from build123d import *

# Parameters (mm, degrees)
F0_R     = 1.8
F0_R_2   = 11.25
F1_DEPTH = 3
F2_W     = 60
F2_H     = 5
F3_DEPTH = 17
F4_R     = 1.8
F5_DEPTH = 5.001
F6_R     = 5
F7_R     = 5


with BuildPart() as f1:
    # F0 (on Front) → F1 (new body)
    with BuildSketch(Plane.XZ):
        Polygon((-21, -21), (21, -21), (21, 21), (21, 31), (-21, 31), (-21, 21), align=None)
        with Locations((-15.7, -15.7)):
            Circle(F0_R, mode=Mode.SUBTRACT)
        with Locations((15.7, -15.7)):
            Circle(F0_R, mode=Mode.SUBTRACT)
        Circle(F0_R_2, mode=Mode.SUBTRACT)
        with Locations((-15.7, 15.7)):
            Circle(F0_R, mode=Mode.SUBTRACT)
        with Locations((15.7, 15.7)):
            Circle(F0_R, mode=Mode.SUBTRACT)
    extrude(amount=F1_DEPTH)

    # F2 (on face) → F3 (join)
    with BuildSketch(Plane.XZ.offset(3)):
        with Locations((0, 28.5)):
            Rectangle(F2_W, F2_H)
    extrude(amount=-F3_DEPTH)

    # F4 (on face) → F5 (cut, through all)
    with BuildSketch(Plane(origin=(0, 0, 26), x_dir=(1, 0, 0), z_dir=(0, 0, -1))):
        with Locations((-21.55957, -7)):
            Circle(F4_R)
        with Locations((21.55957, -7)):
            Circle(F4_R)
    extrude(amount=-F5_DEPTH, mode=Mode.SUBTRACT)

    # F6
    f6_edges = [f1.edges().sort_by_distance(p)[0] for p in [
        (21, -1.5, -21),
        (-21, -1.5, -21),
    ]]
    fillet(f6_edges, radius=F6_R)

    # F7
    f7_edges = [f1.edges().sort_by_distance(p)[0] for p in [
        (-30, -3, 28.5),
        (-30, 14, 28.5),
        (30, -3, 28.5),
        (30, 14, 28.5),
    ]]
    fillet(f7_edges, radius=F7_R)


solid = f1.part
Build history of the part. All positions in model axes, mm. A direction names the side the tool comes from. Coordinates: 2 decimals unless noted, no trailing zeros. Order: outer loops, then holes, each group sorted by start corner. A loop starts at its lowest first (then second) coordinate and runs counter-clockwise, first axis right, second up. Notation, with made-up numbers: M -7.5,-4 L 3.5,-4 A17 ccw 3.5,6 Z; hole C -25,85 d2. An arc over 180 degrees is marked long. One line per question, with ' | ' between items. Start each with the question number.
Q1. Probe L1, parallel to Z at x = 15.7, y = -0.9; L2, parallel to X at y = 7, z = 28.65; L3, parallel to Y at x = 7.5, z = -17. List the from-to ranges inside material, lowest first. Write a range as from..to.
Q2. Flat gauge pins, fed straight in: pin 1 Ø4 at (x, z) = (-22, -11) entering from +Y; pin 2 Ø0.9 at (y, z) = (-1, -3) entering from +X; pin 3 Ø0.9 at (y, z) = (-1, 12) entering from -X. Where does each tip first touch, or does it go through?
Q3. Saw through at B-B (x = 0). List the corners of the cut face in (y, z), then the cut area to 4 significant figures.
Q4. Saw through at C-C (z = 4). List the corners of the cut face in (x, y), then the cut area to 3 significant figures.
Q5. Saw through at D-D (x = -6.5). List the corners of the cut face in (y, z).
Q6. Saw through at A-A (z = 15.7). List the corners of the cut face in (x, y), then the cut area to 3 significant figures.
Q7. Two-plate mould, pull along Z, no slides. Class faces 1 (the face through (-17.128, -1.479, -16.795)), 2 (the face through (28, -2, 29)), 3 (the face through (14.373, -1.479, 16.917)), 4 (the face through (0, 7, 26)): +Z half, -Z half, draft (parallel to the pull), parting line (faces both ways), or undercut.
Q8. 3-axis set-ups, long thin cutter, end or side, ignore diameter. For faces 5 (the face through (21, -1, 5)), 6 (the face through (0, 5, 31)), 7 (the face through (-21, -1, 5)): which of +Z, -Z, +X, -X, +Y, -Y reach the whole face in a straight line?
Check values:
1) L1: z = -21..-17.5, -13.9..13.9, 17.5..31 | L2: x = -30..-23.36, -19.76..19.76, 23.36..30 | L3: y = -3..0
2) pin 1: stops at y = 0 | pin 2: stops at x = 21 | pin 3: stops at x = -21
3) outline: M -3,-21 L 0,-21 L 0,-11.25 L -3,-11.25 Z; M -3,11.25 L 0,11.25 L 0,26 L 14,26 L 14,31 L -3,31 Z | area: 158.5 mm2
4) outline: M -21,-3 L -10.51,-3 L -10.51,0 L -21,0 Z; M 10.51,-3 L 21,-3 L 21,0 L 10.51,0 Z | area: 62.9 mm2
5) outline: M -3,-21 L 0,-21 L 0,-9.18 L -3,-9.18 Z; M -3,9.18 L 0,9.18 L 0,26 L 14,26 L 14,31 L -3,31 Z
6) outline: M -21,-3 L -17.5,-3 L -17.5,0 L -21,0 Z; M -13.9,-3 L 13.9,-3 L 13.9,0 L -13.9,0 Z; M 17.5,-3 L 21,-3 L 21,0 L 17.5,0 Z | area: 104 mm2
7) face 1: undercut | face 2: draft | face 3: undercut | face 4: -Z half
8) face 5: -Z, +X, +Y, -Y | face 6: +Z, +X, -X, +Y, -Y | face 7: -Z, -X, +Y, -Y
